The model under review builds one solid part; all positions refer to its coordinate system, in mm. Face numbers are marked on the shaded views. A direction names the side the tool comes from. Round coordinates to 2 decimals unless told otherwise and drop trailing zeros. Loops run counter-clockwise (first coordinate to the right, second up) from the corner with the lowest first, then second, coordinate; pieces in that order, holes last. Notation, with made-up numbers: (83.25, 58.5) -> (93.25, 58.5) arc R26 cw to (93.25, 87.5) -> close; hole circle Ø7 at (74, 76.5). An arc over 180 degrees is marked (long way). Use a Markdown table: item, result. Add a question column.
1) Consider section B-B on z = -17. Give the boundary of the cut face in (x, y).
2) Consider section D-D on z = 0.75. Give the boundary of the cut face in (x, y).
3) Insertion check: pin 1 (2.5 mm diameter, centred on x = 1, z = -7, fed in from -Y); pin 2 (0.6 mm diameter, centred on x = -4, z = -16.5, fed in from -Y); pin 3 (2 mm diameter, centred on y = -1, z = -15, fed in from -X). Each pin has a flat end and moves straight along its axis. Give the tip position at first contact, or say it passes through.
4) Consider section C-C on y = 0. Give the boundary of the cut face in (x, z), plus the area to 3 significant figures.
5) Wall thickness on probe 1 along Y at (x, z) = (-0.25, -2.75); probe 2 along Y at (x, z) = (-1, -4.25); probe 3 along Z at (x, y) = (-2.25, -1.25): over which ranges is each line inside the solid? List them lowest first.
6) For the marked faces 1, 2, 3 and 4, list the 3-axis set-ups (+Z, -Z, +X, -X, +Y, -Y) from which the entire face can be reached by the end or side of a thin tool; tool diameter is ignored.
7) Mouldability with a two-part tool opening along Z and no side actions: class the marked faces 5, 6 and 7 as released by +Z, released by -Z, zero draft, split by the parting line, or undercut.
8) Consider section A-A on x = 0. Give the boundary of the cut face in (y, z).
from build123d import *

# Parameters (mm, degrees)
SKETCH1_R           = 9.65
BOSS_EXTRUDE1_DEPTH = 2.8
CHAMFER1_SIZE       = 1
SKETCH2_R           = 6.4
BOSS_EXTRUDE2_DEPTH = 3.6
FILLET1_R           = 0.6
SKETCH3_R           = 7.9
BOSS_EXTRUDE3_DEPTH = 13.3
CUT_EXTRUDE1_START  = -13.3
CUT_EXTRUDE1_DEPTH  = 13.3
SKETCH4_W           = 0.8
SKETCH4_H           = 4
BOSS_EXTRUDE4_DEPTH = 5.6
BOSS_EXTRUDE6_DEPTH = 1.8
CIRPATTERN1_COUNT   = 2


with BuildPart() as part:
    # Sketch1 → Boss-Extrude1 (new body)
    with BuildSketch(Plane.XY):
        Circle(SKETCH1_R)
    extrude(amount=BOSS_EXTRUDE1_DEPTH)

    # Chamfer1
    chamfer1_edges = [part.edges().sort_by_distance(p)[0] for p in [
        (-9.65, 0, 2.8),
    ]]
    chamfer(chamfer1_edges, length=CHAMFER1_SIZE)

    # Sketch2 → Boss-Extrude2 (add)
    with BuildSketch(Plane.XY.offset(2.8)):
        Circle(SKETCH2_R)
    extrude(amount=BOSS_EXTRUDE2_DEPTH)

    # Fillet1
    fillet1_edges = [part.edges().sort_by_distance(p)[0] for p in [
        (-6.4, 0, 6.4),
    ]]
    fillet(fillet1_edges, radius=FILLET1_R)

    # Sketch3 → Boss-Extrude3 (add)
    with BuildSketch(Plane(origin=(0, 0, 0), x_dir=(-1, 0, 0), z_dir=(0, 0, -1))):
        Circle(SKETCH3_R)
    extrude(amount=BOSS_EXTRUDE3_DEPTH)

    # Sketch6 → Cut-Extrude1 (cut)
    with BuildSketch(Plane(origin=(0, 0, -13.3), x_dir=(-1, 0, 0), z_dir=(0, 0, -1)).offset(CUT_EXTRUDE1_START)):
        with BuildLine():
            ThreePointArc((2.481934729, 7.5), (0, 7.9), (-2.481934729, 7.5))
            Line((-2.481934729, 7.5), (2.481934729, 7.5))
        make_face()
        with BuildLine():
            Line((2.481934729, -7.5), (-2.481934729, -7.5))
            ThreePointArc((-2.481934729, -7.5), (0, -7.9), (2.481934729, -7.5))
        make_face()
    extrude(amount=CUT_EXTRUDE1_DEPTH, mode=Mode.SUBTRACT)

    # Sketch4 → Boss-Extrude4 (add)
    with BuildSketch(Plane(origin=(0, 0, -13.3), x_dir=(-1, 0, 0), z_dir=(0, 0, -1))):
        with Locations((4.25, 0)):
            Rectangle(SKETCH4_W, SKETCH4_H)
        with Locations((-4.25, 0)):
            Rectangle(SKETCH4_W, SKETCH4_H)
    extrude(amount=BOSS_EXTRUDE4_DEPTH)

    # Sketch8 → Boss-Extrude6 (add, symmetric)
    with BuildSketch(Plane(origin=(0, 0, 0), x_dir=(0, 0, -1), z_dir=(1, 0, 0))):
        Polygon((0, -7.639808061), (0, -8.620963842), (2.146086769, -10.1447862), (9.881224656, -7.5), (7.408497384, -7.5), (2.275068918, -9.2552138), align=None)
    boss_extrude6 = extrude(amount=BOSS_EXTRUDE6_DEPTH, both=True)

    # CirPattern1: Boss-Extrude6 ×2 about axis
    cirpattern1_axis = Axis((0, 0, -13.3), (0, 0, 1))
    for i in range(1, CIRPATTERN1_COUNT):
        add(boss_extrude6.rotate(cirpattern1_axis, i * 360 / CIRPATTERN1_COUNT))


solid = part.part
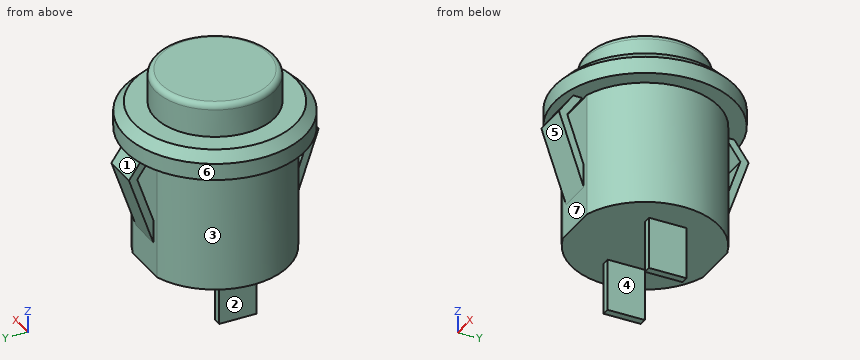
Result set:
| question | item | result |
|---|---|---|
| 1 | outline | (-4.65, -2) -> (-3.85, -2) -> (-3.85, 2) -> (-4.65, 2) -> close; (3.85, -2) -> (4.65, -2) -> (4.65, 2) -> (3.85, 2) -> close |
| 2 | outline | circle Ø19.3 at (0, 0) |
| 3 | pin 1 | y = -8.91 |
| 3 | pin 2 | y = -2 |
| 3 | pin 3 | x = -4.65 |
| 4 | outline | (-9.65, 0) -> (-7.9, 0) -> (-7.9, -13.3) -> (-4.65, -13.3) -> (-4.65, -18.9) -> (-3.85, -18.9) -> (-3.85, -13.3) -> (3.85, -13.3) -> (3.85, -18.9) -> (4.65, -18.9) -> (4.65, -13.3) -> (7.9, -13.3) -> (7.9, 0) -> (9.65, 0) -> (9.65, 1.8) -> (8.65, 2.8) -> (6.4, 2.8) -> (6.4, 5.8) arc R0.6 ccw to (5.8, 6.4) -> (-5.8, 6.4) arc R0.6 ccw to (-6.4, 5.8) -> (-6.4, 2.8) -> (-8.65, 2.8) -> (-9.65, 1.8) -> close |
| 4 | area | 318 mm2 |
| 5 | probe 1 | -9.94 to -9.09, -7.5 to 7.5, 9.09 to 9.94 |
| 5 | probe 2 | -9.43 to -8.58, -7.5 to 7.5, 8.58 to 9.43 |
| 5 | probe 3 | -13.3 to 6.4 |
| 6 | face 1 | +X, -X, +Y |
| 6 | face 2 | -Z, -X, +Y, -Y |
| 6 | face 3 | -Z, -X |
| 6 | face 4 | -Z, +Y, -Y |
| 7 | face 5 | released by -Z |
| 7 | face 6 | zero draft |
| 7 | face 7 | undercut |
| 8 | outline | (-10.14, -2.15) -> (-7.5, -9.88) -> (-7.5, -13.3) -> (7.5, -13.3) -> (7.5, -9.88) -> (10.14, -2.15) -> (8.62, 0) -> (9.65, 0) -> (9.65, 1.8) -> (8.65, 2.8) -> (6.4, 2.8) -> (6.4, 5.8) arc R0.6 ccw to (5.8, 6.4) -> (-5.8, 6.4) arc R0.6 ccw to (-6.4, 5.8) -> (-6.4, 2.8) -> (-8.65, 2.8) -> (-9.65, 1.8) -> (-9.65, 0) -> (-8.62, 0) -> close; hole (-9.26, -2.28) -> (-7.5, -7.41) -> (-7.5, 0) -> (-7.64, 0) -> close; hole (7.5, -7.41) -> (9.26, -2.28) -> (7.64, 0) -> (7.5, 0) -> close |
